```python
from build123d import *

# Parameters (mm, degrees)
F0_W     = 100
F0_H     = 5
F0_W_2   = 5
F0_W_3   = 5.25
F0_H_2   = 4.5
F0_H_3   = 104.3127122521
F0_H_4   = 90.6872877479
F1_DEPTH = 5


with BuildPart() as f1:
    # F0 (on Top) → F1 (new body)
    with BuildSketch(Plane.XY):
        with Locations((50, -2.5)):
            Rectangle(F0_W, F0_H)
        with Locations((102.5, -2.5)):
            Rectangle(F0_W_2, F0_H)
        with Locations((102.5, 2.5)):
            Rectangle(F0_W_2, F0_H)
        with Locations((102.5, -7.5)):
            Rectangle(F0_W_2, F0_H)
        with Locations((107.625, -2.5)):
            Rectangle(F0_W_3, F0_H)
        Polygon((-5, -5), (-5, 0), (-44.7830312261, 0), (-46.2334911863, -2.2172048721), (-44.4696663442, -5), align=None)
        with Locations((-2.5, 111.5627122521)):
            Rectangle(F0_W_2, F0_H_2)
        with Locations((-2.5, 106.8127122521)):
            Rectangle(F0_W_2, F0_H)
        with Locations((-7.5, 106.8127122521)):
            Rectangle(F0_W_2, F0_H)
        with Locations((2.5, 106.8127122521)):
            Rectangle(F0_W_2, F0_H)
        with Locations((-2.5, 52.1563561261)):
            Rectangle(F0_W_2, F0_H_3)
        with Locations((-2.5, -2.5)):
            Rectangle(F0_W_2, F0_H)
        with Locations((-2.5, -50.3436438739)):
            Rectangle(F0_W_2, F0_H_4)
        Polygon((-46.2334911863, -2.2172048721), (-44.7830312261, 0), (-46.8160055033, 0), (-47.3614148705, -0.862929156), (-47.9020566732, 0), (-50.0197165479, 0), (-48.535376256, -2.2862614242), (-50.2615776366, -5), (-48.1912470634, -5), (-47.4074525719, -3.7402854932), (-46.6374528634, -5), (-44.4696663442, -5), align=None)
        Polygon((-46.8160055033, 0), (-44.7830312261, 0), (-40.8048788968, 6.0810908044), (-42.9724873375, 6.0810908044), align=None)
        with Locations((-2.5, -98.1872877479)):
            Rectangle(F0_W_2, F0_H)
        with Locations((-7.5, -98.1872877479)):
            Rectangle(F0_W_2, F0_H)
        Polygon((-40.382866634, -11.4477640018), (-44.4696663442, -5), (-46.6374528634, -5), (-42.6962611291, -11.4477640018), align=None)
        Polygon((-47.3614148705, -0.862929156), (-46.8160055033, 0), (-47.9020566732, 0), align=None)
        with Locations((2.5, -98.1872877479)):
            Rectangle(F0_W_2, F0_H)
        with Locations((-2.5, -102.9372877479)):
            Rectangle(F0_W_2, F0_H_2)
        Polygon((-48.1912470634, -5), (-46.6374528634, -5), (-47.4074525719, -3.7402854932), align=None)
        Polygon((-50.0197165479, 0), (-47.9020566732, 0), (-51.7119776523, 6.0810908044), (-53.9678250207, 6.0810908044), align=None)
        Polygon((-52.2030464672, -11.4477640018), (-48.1912470634, -5), (-50.2615776366, -5), (-54.3629819576, -11.4477640018), align=None)
        Polygon((-48.535376256, -2.2862614242), (-50.0197165479, 0), (-100, 0), (-100, -5), (-50.2615776366, -5), align=None)
        with Locations((-102.5, -2.5)):
            Rectangle(F0_W_2, F0_H)
        with Locations((-102.5, 2.5)):
            Rectangle(F0_W_2, F0_H)
        with Locations((-102.5, -7.5)):
            Rectangle(F0_W_2, F0_H)
        with Locations((-107.625, -2.5)):
            Rectangle(F0_W_3, F0_H)
    extrude(amount=F1_DEPTH)


solid = f1.part
```
Here's how the part is built. I have some questions about the finished solid (model axes, mm). A direction names the side the tool comes from. Give positions to 0.01 mm unless a question says otherwise; leave off trailing zeros. Loops run counter-clockwise (first coordinate to the right, second up) from the corner with the lowest first, then second, coordinate; pieces in that order, holes last. Notation, with made-up numbers: M -12,42.25 L 1,42.25 A37 cw 1,78.25 Z; hole C 35.5,87 d6. An arc over 180 degrees is marked long. Put each result on its own line as item: value. Start each with the question number.
(1) For faces 1 (the flat face through (-10, -98, 2)), 2 (the flat face through (-10, 107, 2)), 3 (the flat face through (108, -5, 2)), which set-ups out of +Z, -Z, +X, -X, +Y, -Y let a thin tool reach every point of the face, with its end or its side?
(2) Will these pins go through, and if not, where does the flat tip stop? pin 1 Ø2 at (x, z) = (-63, 2.5) entering from -Y; pin 2 Ø2 at (y, z) = (-103, 1.5) entering from -X; pin 3 Ø1.1 at (x, z) = (-53.5, 3) entering from -Y.
(3) I need wall thicknesses on line 1 along Y through (x, z) = (-69, 1.25). Which ranges of the line are inside material? Lowest first, please. Write a range as [from, to].
(4) I want a section at A-A on x = -86.5. Please give me the cut outline in (y, z).
Answer block:
1. face 1: +Z, -Z, -X, -Y
1. face 2: +Z, -Z, -X, +Y
1. face 3: +Z, -Z, +X, -Y
2. pin 1: y = -5
2. pin 2: x = -5
2. pin 3: y = -11.45
3. line 1: [-5, 0]
4. outline: M -5,0 L 0,0 L 0,5 L -5,5 Z
